Geometry check sheet. Reference: the model listing, model coordinates, mm. Give positions to 0.01 mm unless a question says otherwise; leave off trailing zeros. Loops run counter-clockwise (first coordinate to the right, second up) from the corner with the lowest first, then second, coordinate; pieces in that order, holes last. Notation, with made-up numbers: (10, 58) - (34, 58) arc R26 cw to (34, 74) - close; hole circle Ø5 at (74, 14). An arc over 180 degrees is marked (long way). Write item = value, one per line. Start each with the question number.
Autodesk Fusion 360 part; units mm, degrees
sketch "Sketch1" plane through (0, 0, 0) normal (0, 1, 0) x (1, 0, 0)
  line L0 (0, 0) -> (149, 0)
  line L1 (149, 0) -> (149, -107)
  line L2 (0, 0) -> (0, -107)
  line L3 (0, -107) -> (149, -107)
  line L4 (0, -107) -> (0, -115.3)
  line L5 (0, -115.3) -> (8, -115.3)
  line L6 (8, -115.3) -> (8, -107)
  line L7 (149, -107) -> (149, -115.3)
  line L8 (149, -115.3) -> (141, -115.3)
  line L9 (141, -115.3) -> (141, -107)
  line L10 (141, -107) -> (149, -115.3) construction
  line L11 (141, -115.3) -> (149, -107) construction
  circle A0 centre (145, -111.15) radius 0.75
  circle A1 centre (4, -111.15) radius 0.75
  line L12 (0, -115.3) -> (8, -107) construction
  line L13 (8, -115.3) -> (0, -107) construction
  line L14 (0, 0) -> (0, 8.3)
  line L15 (0, 8.3) -> (8, 8.3)
  line L16 (8, 8.3) -> (8, 0)
  line L17 (149, 0) -> (149, 8.3)
  line L18 (149, 8.3) -> (141, 8.3)
  line L19 (141, 8.3) -> (141, 0)
  line L20 (149, 0) -> (141, 8.3) construction
  line L21 (141, 0) -> (149, 8.3) construction
  line L22 (0, 0) -> (8, 8.3) construction
  line L23 (8, 0) -> (0, 8.3) construction
  circle A2 centre (4, 4.15) radius 0.75
  circle A3 centre (145, 4.15) radius 0.75
  dimension "d1" = 149
  dimension "d2" = 107
  dimension "d3" = 107
  dimension "d4" = 149
  dimension "d5" = 8.3
  dimension "d6" = 8
  dimension "d7" = 8.3
  dimension "d8" = 8
  dimension "d9" = 1.5
  dimension "d10" = 1.5
  dimension "d11" = 8.3
  dimension "d12" = 8
  dimension "d13" = 8.3
  dimension "d14" = 8
  dimension "d15" = 1.5
  dimension "d16" = 1.5
extrude "Extrude1" add sketch "Sketch1" against normal blind 1.65
sketch "Sketch2" plane through (0, -1.65, 0) normal (0, -1, 0) x (1, 0, 0)
  circle A0 centre (145, -4.15) radius 0.75
  circle A1 centre (4, 111.15) radius 0.75
  circle A2 centre (145, 111.15) radius 0.75
  circle A3 centre (4, -4.15) radius 0.75
  line L0 (149, -8.3) -> (149, 115.3)
  line L1 (149, 115.3) -> (141, 115.3)
  line L2 (141, 115.3) -> (141, 107)
  line L3 (141, 107) -> (8, 107)
  line L4 (8, 107) -> (8, 115.3)
  line L5 (8, 115.3) -> (0, 115.3)
  line L6 (0, 115.3) -> (0, -8.3)
  line L7 (0, -8.3) -> (8, -8.3)
  line L8 (8, -8.3) -> (8, 0)
  line L9 (8, 0) -> (141, 0)
  line L10 (141, 0) -> (141, -8.3)
  line L11 (141, -8.3) -> (149, -8.3)
  line L12 (0, 107) -> (0, 103.4) construction
  line L13 (0, 103.4) -> (149, 103.4)
  line L14 (0, 0) -> (0, 3.6) construction
  line L15 (8, 107) -> (-0.0006, 107) construction
  line L16 (8, 0) -> (0, 0) construction
  line L17 (0, 3.6) -> (149, 3.6)
  dimension "d19" = 3.6
  dimension "d20" = 3.6
extrude "Extrude2" add sketch "Sketch2" along normal blind 6.3 contours L0 L6 L13 L17
sketch "Sketch3" plane through (149, 0, 0) normal (1, 0, 0) x (0, 1, 0)
  line L0 (0, -8.3) -> (0, 115.3)
  line L1 (0, 115.3) -> (-1.65, 115.3)
  line L2 (-1.65, 115.3) -> (-1.65, 103.4)
  line L3 (-1.65, 103.4) -> (-7.95, 103.4)
  line L4 (-7.95, 103.4) -> (-7.95, 3.6)
  line L5 (-7.95, 3.6) -> (-1.65, 3.6)
  line L6 (-1.65, 3.6) -> (-1.65, -8.3)
  line L7 (-1.65, -8.3) -> (0, -8.3)
sketch "Sketch4" plane through (0, 0, 0) normal (0, 1, 0) x (-1, 0, 0)
  circle A0 centre (-145, -4.15) radius 0.75
  circle A1 centre (-4, 111.15) radius 0.75
  circle A2 centre (-145, 111.15) radius 0.75
  circle A3 centre (-4, -4.15) radius 0.75
  line L0 (-149, 115.3) -> (-149, -8.3)
  line L1 (-149, -8.3) -> (-141, -8.3)
  line L2 (-141, -8.3) -> (-141, 0)
  line L3 (-141, 0) -> (-8, 0)
  line L4 (-8, 0) -> (-8, -8.3)
  line L5 (-8, -8.3) -> (0, -8.3)
  line L6 (0, -8.3) -> (0, 115.3)
  line L7 (0, 115.3) -> (-8, 115.3)
  line L8 (-8, 115.3) -> (-8, 107)
  line L9 (-8, 107) -> (-141, 107)
  line L10 (-141, 107) -> (-141, 115.3)
  line L11 (-141, 115.3) -> (-149, 115.3)
  line L12 (-149, 106.8976) -> (-149, 86.2976) construction
  line L13 (-149, 86.2976) -> (-137, 86.2976)
  line L14 (-137, 86.2976) -> (-137, 71.0976)
  line L15 (-137, 71.0976) -> (-149, 71.0976)
  dimension "d23" = 20.6
  dimension "d24" = 12
  dimension "d25" = 15.2
extrude "Extrude3" add sketch "Sketch4" along normal blind 5.6 contours L0 L13 L14 L15
sketch "Sketch5" plane through (149, 0, 0) normal (1, 0, 0) x (0, 1, 0)
  line L0 (0, -8.3) -> (0, 71.0976)
  line L1 (0, 71.0976) -> (5.6, 71.0976)
  line L2 (5.6, 71.0976) -> (5.6, 86.2976)
  line L3 (5.6, 86.2976) -> (0, 86.2976)
  line L4 (0, 86.2976) -> (0, 115.3)
  line L5 (0, 115.3) -> (-1.65, 115.3)
  line L6 (-1.65, 115.3) -> (-1.65, 103.4)
  line L7 (-1.65, 103.4) -> (-7.95, 103.4)
  line L8 (-7.95, 103.4) -> (-7.95, 3.6)
  line L9 (-7.95, 3.6) -> (-1.65, 3.6)
  line L10 (-1.65, 3.6) -> (-1.65, -8.3)
  line L11 (-1.65, -8.3) -> (0, -8.3)
  line L12 (0, 86.2976) -> (0, 71.0976)
  line L13 (0, 86.2976) -> (0, 85.5476) construction
  arc A0 (0, 85.5476) -> (1.1901, 86.2976) centre (0.2339, 86.4956) ccw
  line L14 (0, 71.0976) -> (0, 71.8476) construction
  arc A1 (1.4983, 71.0976) -> (0, 71.8476) centre (0.1697, 70.3149) ccw
  dimension "d29" = 0.75
  dimension "d30" = 0.75
extrude "Extrude4" cut sketch "Sketch5" against normal blind 4 contours L1 L12 A1 | L3 L12 A0
sketch "Sketch6" plane through (149, 0, 0) normal (1, 0, 0) x (0, 1, 0)
  arc A0 (0, 85.5476) -> (1.1901, 86.2976) centre (0.2339, 86.4956) ccw
  line L0 (0, 85.5476) -> (0, 115.3)
  line L1 (0, 115.3) -> (-1.65, 115.3)
  line L2 (-1.65, 115.3) -> (-1.65, 103.4)
  line L3 (-1.65, 103.4) -> (-7.95, 103.4)
  line L4 (-7.95, 103.4) -> (-7.95, 3.6)
  line L5 (-7.95, 3.6) -> (-1.65, 3.6)
  line L6 (-1.65, 3.6) -> (-1.65, -8.3)
  line L7 (-1.65, -8.3) -> (0, -8.3)
  line L8 (0, -8.3) -> (0, 71.8476)
  arc A1 (1.4983, 71.0976) -> (0, 71.8476) centre (0.1697, 70.3149) ccw
  line L9 (1.4983, 71.0976) -> (5.6, 71.0976)
  line L10 (5.6, 71.0976) -> (5.6, 86.2976)
  line L11 (5.6, 86.2976) -> (1.1901, 86.2976)
  line L12 (1, 85) -> (1, 73)
  line L13 (1, 73) -> (4, 73)
  line L14 (4, 73) -> (4, 85)
  line L15 (4, 85) -> (1, 85)
extrude "Extrude5" cut sketch "Sketch6" against normal blind 10 contours L12 L13 L14 L15
sketch "Sketch7" plane through (0, 0, 86.2976) normal (0, 0, 1) x (-1, 0, 0)
  line L0 (-145, 0) -> (-145, -1.1901)
  line L1 (-145, -1.1901) -> (-149, -1.1901)
  line L2 (-149, -1.1901) -> (-149, -5.6)
  line L3 (-149, -5.6) -> (-137, -5.6)
  line L4 (-137, -5.6) -> (-137, 0)
  line L5 (-137, 0) -> (-145, 0)
sketch "Sketch8" plane through (0, 0, 0) normal (0, 1, 0) x (-1, 0, 0)
  line L0 (-137, 71.0976) -> (-145, 71.0976)
  line L1 (-145, 71.0976) -> (-145, 71.8476)
  line L2 (-145, 71.8476) -> (-149, 71.8476)
  line L3 (-149, 71.8476) -> (-149, -8.3)
  line L4 (-149, -8.3) -> (-141, -8.3)
  line L5 (-141, -8.3) -> (-141, 0)
  line L6 (-141, 0) -> (-8, 0)
  line L7 (-8, 0) -> (-8, -8.3)
  line L8 (-8, -8.3) -> (0, -8.3)
  line L9 (0, -8.3) -> (0, 115.3)
  line L10 (0, 115.3) -> (-8, 115.3)
  line L11 (-8, 115.3) -> (-8, 107)
  line L12 (-8, 107) -> (-141, 107)
  line L13 (-141, 107) -> (-141, 115.3)
  line L14 (-141, 115.3) -> (-149, 115.3)
  line L15 (-149, 115.3) -> (-149, 85.5476)
  line L16 (-149, 85.5476) -> (-145, 85.5476)
  line L17 (-145, 85.5476) -> (-145, 86.2976)
  line L18 (-145, 86.2976) -> (-137, 86.2976)
  line L19 (-137, 86.2976) -> (-137, 71.0976)
  circle A0 centre (-145, -4.15) radius 0.75
  circle A1 centre (-4, 111.15) radius 0.75
  circle A2 centre (-145, 111.15) radius 0.75
  circle A3 centre (-4, -4.15) radius 0.75
  line L20 (-149, 71.0976) -> (-149, 62.1976) construction
  line L21 (-149, 62.1976) -> (-143.7, 62.1976)
  line L22 (-143.7, 62.1976) -> (-143.7, 54.5976)
  line L23 (-143.7, 54.5976) -> (-149, 54.5976)
  dimension "d35" = 8.9
  dimension "d36" = 5.3
  dimension "d37" = 7.6
extrude "Extrude6" add sketch "Sketch8" along normal blind 2.75 contours L3 L21 L22 L23
sketch "Sketch9" plane through (149, 0, 0) normal (1, 0, 0) x (0, 1, 0)
  line L0 (1, 73) -> (1, 85)
  line L1 (1, 85) -> (4, 85)
  line L2 (4, 85) -> (4, 73)
  line L3 (4, 73) -> (1, 73)
  arc A0 (0, 85.5476) -> (1.1901, 86.2976) centre (0.2339, 86.4956) ccw
  line L4 (0, 85.5476) -> (0, 115.3)
  line L5 (0, 115.3) -> (-1.65, 115.3)
  line L6 (-1.65, 115.3) -> (-1.65, 103.4)
  line L7 (-1.65, 103.4) -> (-7.95, 103.4)
  line L8 (-7.95, 103.4) -> (-7.95, 3.6)
  line L9 (-7.95, 3.6) -> (-1.65, 3.6)
  line L10 (-1.65, 3.6) -> (-1.65, -8.3)
  line L11 (-1.65, -8.3) -> (0, -8.3)
  line L12 (0, -8.3) -> (0, 54.5976)
  line L13 (0, 54.5976) -> (2.75, 54.5976)
  line L14 (2.75, 54.5976) -> (2.75, 62.1976)
  line L15 (2.75, 62.1976) -> (0, 62.1976)
  line L16 (0, 62.1976) -> (0, 71.8476)
  arc A1 (1.4983, 71.0976) -> (0, 71.8476) centre (0.1697, 70.3149) ccw
  line L17 (1.4983, 71.0976) -> (5.6, 71.0976)
  line L18 (5.6, 71.0976) -> (5.6, 86.2976)
  line L19 (5.6, 86.2976) -> (1.1901, 86.2976)
  line L20 (2.75, 62.1976) -> (0, 61.5)
  line L21 (2.75, 62.1976) -> (0, 61.5)
  line L22 (2.75, 54.5976) -> (0, 55.2952)
  line L23 (0, 62.1976) -> (0, 61.5)
  line L24 (0, 55.2952) -> (0, 54.5976)
extrude "Extrude7" cut sketch "Sketch9" against normal blind 1.1 contours L15 L20 L21 L23 | L13 L22 L24
sketch "Sketch10" plane through (149, 0, 0) normal (1, 0, 0) x (0, 1, 0)
  line L0 (1, 73) -> (1, 85)
  line L1 (1, 85) -> (4, 85)
  line L2 (4, 85) -> (4, 73)
  line L3 (4, 73) -> (1, 73)
  line L4 (0, -8.3) -> (0, 55.2952)
  line L5 (0, 55.2952) -> (2.75, 54.5976)
  line L6 (2.75, 54.5976) -> (2.75, 62.1976)
  line L7 (2.75, 62.1976) -> (0, 61.5)
  line L8 (0, 61.5) -> (0, 71.8476)
  arc A0 (1.4983, 71.0976) -> (0, 71.8476) centre (0.1697, 70.3149) ccw
  line L9 (1.4983, 71.0976) -> (5.6, 71.0976)
  line L10 (5.6, 71.0976) -> (5.6, 86.2976)
  line L11 (5.6, 86.2976) -> (1.1901, 86.2976)
  arc A1 (0, 85.5476) -> (1.1901, 86.2976) centre (0.2339, 86.4956) ccw
  line L12 (0, 85.5476) -> (0, 115.3)
  line L13 (0, 115.3) -> (-1.65, 115.3)
  line L14 (-1.65, 115.3) -> (-1.65, 103.4)
  line L15 (-1.65, 103.4) -> (-7.95, 103.4)
  line L16 (-7.95, 103.4) -> (-7.95, 3.6)
  line L17 (-7.95, 3.6) -> (-1.65, 3.6)
  line L18 (-1.65, 3.6) -> (-1.65, -8.3)
  line L19 (-1.65, -8.3) -> (0, -8.3)
  line L20 (0.3, 61) -> (2.4, 61)
  line L21 (2.4, 61) -> (2.4, 55.5)
  line L22 (2.4, 55.5) -> (0.5, 55.5)
  line L23 (0.5, 55.5) -> (0.3, 55.5)
  line L24 (0.3, 55.5) -> (0.3, 61)
extrude "Extrude8" cut sketch "Sketch10" against normal blind 4.1 contours L20 L21 L22 L23 L24
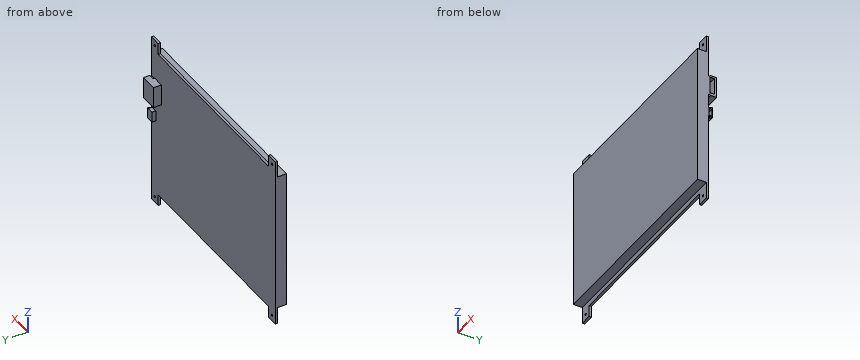
1) Gauge pin test, flat ends, axial feed: P1, Ø2, axis at y = 1.5, z = 58, coming from the -X side; P2, Ø0.9, axis at x = 4, z = -4.15, coming from the +Y side; P3, Ø1.5, axis at x = 145.5, y = 2, coming from the +Z side; P4, Ø1.5, axis at x = 112, z = 95.5, coming from the +Y side. Record the tip position at first contact, or that the pin passes through.
2) Cross-section at C-C on y = -6. Enter the section's corners in (x, z), and give its area (3 significant figures).
3) Cross-section at A-A on z = 80.5. Enter the section's corners in (x, y).
4) Material ranges on line 1 along X through (y, z) = (-1, 111.15); line 2 along Z through (x, y) = (145, -0.45); line 3 along Y through (x, z) = (125, 96.5), recorded low to high.
5) Cross-section at B-B on x = 109. Enter the section's corners in (y, z), and give its area (3 significant figures).
6) Cross-section at D-D on z = 94.5. Enter the section's corners in (x, y).
Checked values:
q1.P1 = 143.7
q1.P2 = through
q1.P3 = 86.3
q1.P4 = 0
q2.outline = (0, 3.6) - (149, 3.6) - (149, 103.4) - (0, 103.4) - close
q2.area = 14,900 mm²
q3.outline = (0, -7.95) - (149, -7.95) - (149, 1) - (139, 1) - (139, 4) - (149, 4) - (149, 5.6) - (137, 5.6) - (137, 0) - (0, 0) - close
q4.line_1 = 0 to 3.25, 4.75 to 8, 141 to 144.25, 145.75 to 149
q4.line_2 = -8.3 to -4.9, -3.4 to 110.4, 111.9 to 115.3
q4.line_3 = -7.95 to 0
q5.outline = (-7.95, 3.6) - (-1.65, 3.6) - (-1.65, 0) - (0, 0) - (0, 107) - (-1.65, 107) - (-1.65, 103.4) - (-7.95, 103.4) - close
q5.area = 805 mm²
q6.outline = (0, -7.95) - (149, -7.95) - (149, 0) - (0, 0) - close
